from build123d import *

# Parameters (mm, degrees)
BOSS_EXTRUDE1_DEPTH = 25.4
BOSS_EXTRUDE2_DEPTH = 57.15
FILLET1_R           = 2.54


with BuildPart() as part:
    # Sketch2 → Boss-Extrude1 (new body)
    with BuildSketch(Plane(origin=(0, 0, 0), x_dir=(1, 0, 0), z_dir=(0, 1, 0))):
        Polygon((-56.661538462, 0), (70.338461538, 0), (97.279229902, 26.940768363), (97.279229902, 153.940768363), (70.338461538, 180.881536726), (-56.661538462, 180.881536726), (-83.602306825, 153.940768363), (-83.602306825, 26.940768363), align=None)
    extrude(amount=BOSS_EXTRUDE1_DEPTH)

    # Sketch3 → Boss-Extrude2 (add)
    with BuildSketch(Plane(origin=(0, 25.4, 0), x_dir=(1, 0, 0), z_dir=(0, 1, 0))):
        Polygon((-59.472306825, 36.935741623), (-46.666565201, 24.13), (60.343488278, 24.13), (73.149229902, 36.935741623), (73.149229902, 143.945795103), (60.343488278, 156.751536726), (-46.666565201, 156.751536726), (-59.472306825, 143.945795103), align=None)
    extrude(amount=BOSS_EXTRUDE2_DEPTH)

    # Fillet1
    fillet1_edges = [part.edges().sort_by_distance(p)[0] for p in [
        (-59.472306825, 25.4, -90.440768363),
        (-59.472306825, 53.975, -143.945795103),
        (-53.069436013, 25.4, -30.532870812),
        (-59.472306825, 53.975, -36.935741623),
        (6.838461538, 25.4, -24.13),
        (-46.666565201, 53.975, -24.13),
        (66.74635909, 25.4, -30.532870812),
        (60.343488278, 53.975, -24.13),
        (73.149229902, 25.4, -90.440768363),
        (73.149229902, 53.975, -36.935741623),
        (66.74635909, 25.4, -150.348665915),
        (73.149229902, 53.975, -143.945795103),
        (6.838461538, 25.4, -156.751536726),
        (60.343488278, 53.975, -156.751536726),
        (-53.069436013, 25.4, -150.348665915),
        (-46.666565201, 53.975, -156.751536726),
        (-59.472306825, 82.55, -90.440768363),
        (-53.069436013, 82.55, -30.532870812),
        (6.838461538, 82.55, -24.13),
        (66.74635909, 82.55, -30.532870812),
        (73.149229902, 82.55, -90.440768363),
        (66.74635909, 82.55, -150.348665915),
        (6.838461538, 82.55, -156.751536726),
        (-53.069436013, 82.55, -150.348665915),
    ]]
    fillet(fillet1_edges, radius=FILLET1_R)


solid = part.part
Source: CAD feature listing. Evaluate the final solid. Frame: model axes, mm. A direction names the side the tool comes from. Coordinates: 2 decimals unless noted, no trailing zeros. Write each loop counter-clockwise with the first axis right and the second up, starting at its lowest first coordinate (ties: lowest second). Pieces come first, ordered by that corner, then holes. Notation, with made-up numbers: M -22,14.5 L 0,14.5 A35 cw 0,51.5 Z; hole C 69,-20.5 d1. An arc over 180 degrees is marked long. Use a Markdown table: item, result.
1) Section A-A, the plane z = -91.5. Output: boundary loops of the cut face in (x, y), then the cut area to 3 significant figures.
Conclusion:
| item | result |
|---|---|
| outline | M -83.6,0 L 97.28,0 L 97.28,25.4 L 75.69,25.4 A2.54 cw 73.15,27.94 L 73.15,80.01 A2.54 ccw 70.61,82.55 L -56.93,82.55 A2.54 ccw -59.47,80.01 L -59.47,27.94 A2.54 cw -62.01,25.4 L -83.6,25.4 Z |
| area | 12,200 mm^2 |
2) Section B-B, the plane x = -11. Output: boundary loops of the cut face in (y, z), then the cut area to 3 significant figures.
Conclusion:
| item | result |
|---|---|
| outline | M 0,-180.88 L 25.4,-180.88 L 25.4,-159.29 A2.54 cw 27.94,-156.75 L 80.01,-156.75 A2.54 ccw 82.55,-154.21 L 82.55,-26.67 A2.54 ccw 80.01,-24.13 L 27.94,-24.13 A2.54 cw 25.4,-21.59 L 25.4,0 L 0,0 Z |
| area | 12,200 mm^2 |
3) Section C-C, the plane y = 22.5. Output: boundary loops of the cut face in (x, z), then the cut area to 3 significant figures.
Conclusion:
| item | result |
|---|---|
| outline | M -83.6,-153.94 L -56.66,-180.88 L 70.34,-180.88 L 97.28,-153.94 L 97.28,-26.94 L 70.34,0 L -56.66,0 L -83.6,-26.94 Z |
| area | 31,300 mm^2 |
4) Ray query, L1, parallel to Y at x = -59.5, z = -31; L2, parallel to Z at x = 24.5, y = 38; L3, parallel to X at y = 76, z = -39.5. Return the intervals inside material, ascending.
Conclusion:
| item | result |
|---|---|
| L1 | y = 0 to 25.4 |
| L2 | z = -156.75 to -24.13 |
| L3 | x = -59.47 to 73.15 |
5) Section D-D, the plane y = 38. Output: boundary loops of the cut face in (x, z), then the cut area to 3 significant figures.
Conclusion:
| item | result |
|---|---|
| outline | M -59.47,-142.89 A2.54 ccw -58.73,-144.69 L -47.41,-156.01 A2.54 ccw -45.61,-156.75 L 59.29,-156.75 A2.54 ccw 61.09,-156.01 L 72.41,-144.69 A2.54 ccw 73.15,-142.89 L 73.15,-37.99 A2.54 ccw 72.41,-36.19 L 61.09,-24.87 A2.54 ccw 59.29,-24.13 L -45.61,-24.13 A2.54 ccw -47.41,-24.87 L -58.73,-36.19 A2.54 ccw -59.47,-37.99 Z |
| area | 17,300 mm^2 |
6) Reachability of faces 1 (the flat face through (66.826, 53.611, -150.269)), 2 (the flat face through (-53.149, 53.611, -30.612)), 3 (the flat face through (-52.99, 53.61, -150.43)), 4 (the flat face through (8, 54, -156.752)), 5 (the flat face through (6, 25.4, -165)) from +Z, -Z, +X, -X, +Y, -Y: full face, straight path, thin tool, end or side. Return the list, or none.
Conclusion:
| item | result |
|---|---|
| face 1 | -Z, +X, +Y |
| face 2 | +Z, -X, +Y |
| face 3 | -Z, -X, +Y |
| face 4 | -Z, +X, -X, +Y |
| face 5 | +Y |
7) First-contact query: pin 1 Ø12 at (x, y) = (73.5, 44.5) entering from +Z; pin 2 Ø1 at (x, y) = (5.5, 34) entering from -Z; pin 3 Ø1.5 at (y, z) = (11, -155) entering from +X. Flat tips, straight axial feed; report the tip coordinate or a pass-through.
Conclusion:
| item | result |
|---|---|
| pin 1 | stops at z = -31.29 |
| pin 2 | stops at z = -156.75 |
| pin 3 | stops at x = 96.97 |
